Job drawing, mm, ordinate dimensions from the low corner. One solid piece. A direction names the side the tool comes from. Coordinates: 2 decimals unless noted, no trailing zeros. Order: outer loops, then holes, each group sorted by start corner. A loop starts at its lowest first (then second) coordinate and runs counter-clockwise, first axis right, second up. Notation, with made-up numbers: (71, 86.5) - (98, 86.5) arc R14 ccw to (98, 104.5) - close; hole circle Ø7 at (-5.75, 10). An arc over 180 degrees is marked (long way). Use a Markdown table: item, result. Add a question column.
1) Saw through at C-C on x = 13.25. List the corners of the cut face in (y, z), then the cut area to 3 significant figures.
2) Wall check: L1, parallel to X at y = 13.5, z = 9; L2, parallel to Y at x = 5.5, z = 5; L3, parallel to Z at x = 4.5, y = 18. Give the ranges that are in metal, low to high. Write a range as [from, to].
3) Saw through at B-B on z = 10. List the corners of the cut face in (x, y), then the cut area to 3 significant figures.
4) Saw through at D-D on z = 7.5. List the corners of the cut face in (x, y), then the cut area to 3 significant figures.
5) Saw through at A-A on x = 5.5. List the corners of the cut face in (y, z).
6) Tool access for the marked faces 1, 2 and 3: list every direction of +Z, -Z, +X, -X, +Y, -Y with a clear straight run to the whole face (end or side of a thin tool).
7) Drop flat-ended pins along their axis: P1, Ø12, axis at y = 13, z = 4, coming from the +X side; P2, Ø4, axis at x = 6, y = 3, coming from the -Z side; P3, Ø6, axis at y = 7, z = 9.5, coming from the +X side. Give the stop position or say it passes through.
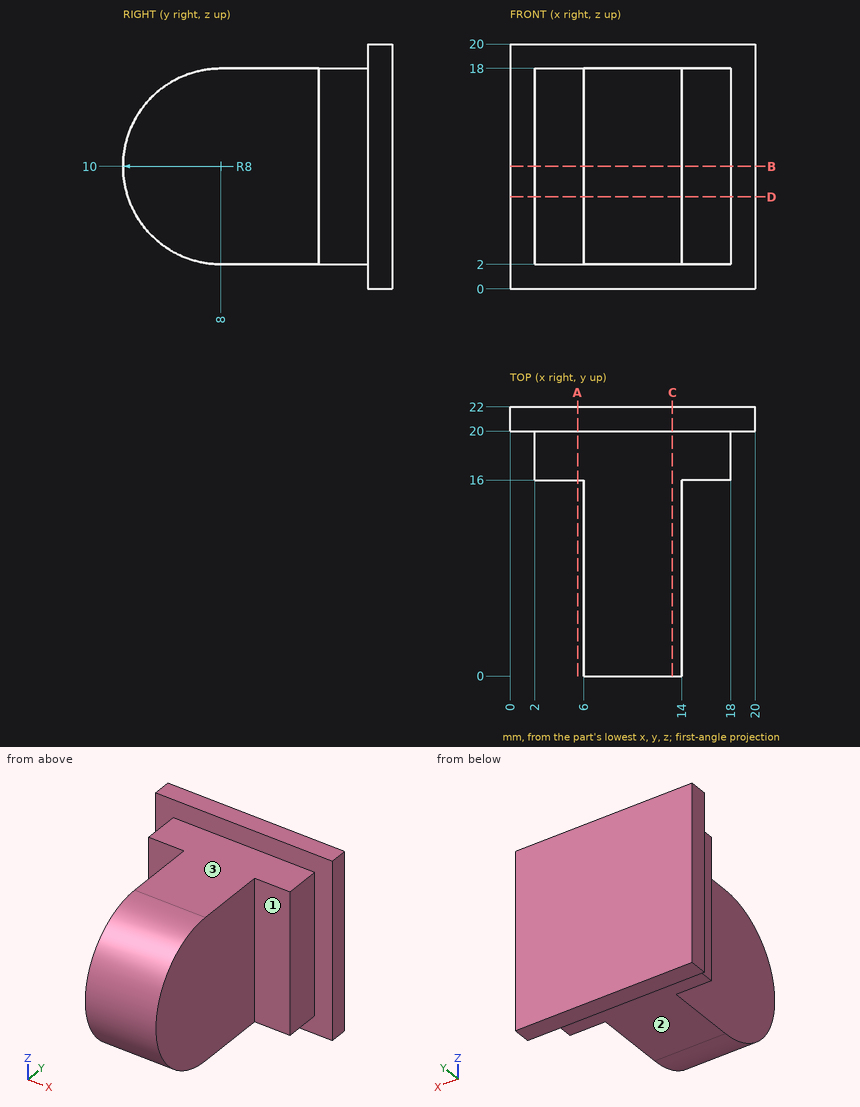
Results are:
| question | item | result |
|---|---|---|
| 1 | outline | (8, 2) - (20, 2) - (20, 0) - (22, 0) - (22, 20) - (20, 20) - (20, 18) - (8, 18) arc R8 ccw to start |
| 1 | area | 333 mm2 |
| 2 | L1 | [6, 14] |
| 2 | L2 | [16, 22] |
| 2 | L3 | [2, 18] |
| 3 | outline | (0, 20) - (2, 20) - (2, 16) - (6, 16) - (6, 0) - (14, 0) - (14, 16) - (18, 16) - (18, 20) - (20, 20) - (20, 22) - (0, 22) - close |
| 3 | area | 232 mm2 |
| 4 | outline | (0, 20) - (2, 20) - (2, 16) - (6, 16) - (6, 0.4) - (14, 0.4) - (14, 16) - (18, 16) - (18, 20) - (20, 20) - (20, 22) - (0, 22) - close |
| 4 | area | 229 mm2 |
| 5 | outline | (16, 2) - (20, 2) - (20, 0) - (22, 0) - (22, 20) - (20, 20) - (20, 18) - (16, 18) - close |
| 6 | face 1 | +Z, -Z, +X, -Y |
| 6 | face 2 | -Z, +X, -X, -Y |
| 6 | face 3 | +Z, +X, -X, -Y |
| 7 | P1 | x = 18 |
| 7 | P2 | z = 2.58 |
| 7 | P3 | x = 14 |
